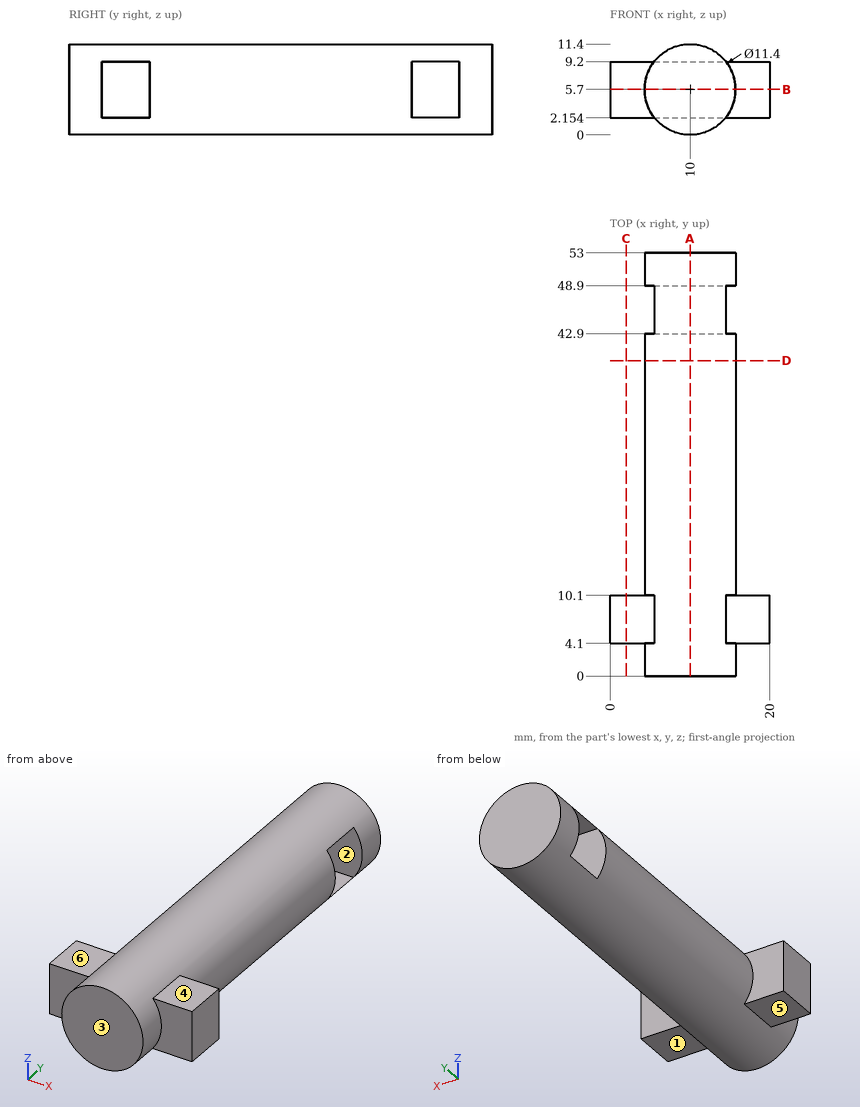
Part print with two shaded views. Sizes in mm from the minimum x, y, z corner. A direction names the side the tool comes from. Give positions to 0.01 mm unless a question says otherwise; leave off trailing zeros. Order: outer loops, then holes, each group sorted by start corner. A loop starts at its lowest first (then second) coordinate and runs counter-clockwise, first axis right, second up. Notation, with made-up numbers: (86.5, 19.5) - (123.5, 19.5) arc R11 ccw to (123.5, 35.5) - close; hole circle Ø2 at (-22.5, 44.25). An arc over 180 degrees is marked (long way). Write each question's results on one line, items separated by ' | '.
1. 3-axis set-ups, long thin cutter, end or side, ignore diameter. For the marked faces 4, 5 and 6: which of +Z, -Z, +X, -X, +Y, -Y reach the whole face in a straight line?
Calculated:
face 4: +Z, +X, +Y, -Y | face 5: -Z, -X, +Y, -Y | face 6: +Z, -X, +Y, -Y
2. Saw through at D-D on y = 39.5. List the corners of the cut face in (x, z), and give its area (3 significant figures).
Calculated:
outline: circle Ø11.4 at (10, 5.7) | area: 102 mm2
3. Pin check, flat tips, straight feed: pin 1 (4.5 mm diameter, centred on x = 4, y = 7, fed in from +Z); pin 2 (6 mm diameter, centred on y = 46.5, z = 7.5, fed in from +X); pin 3 (1.8 mm diameter, centred on x = 8, y = 44.5, fed in from -Z). Stop position of each tip, or through.
Calculated:
pin 1: stops at z = 9.99 | pin 2: stops at x = 15.7 | pin 3: stops at z = 0.11
4. Saw through at C-C on x = 2. List the corners of the cut face in (y, z) (1 decimal).
Calculated:
outline: (4.1, 2.2) - (10.1, 2.2) - (10.1, 9.2) - (4.1, 9.2) - close
5. Pull direction Z, two halves, no side cores. Call the marked faces 1, 2 and 3: released by +Z, released by -Z, zero draft, split by the parting line, or undercut.
Calculated:
face 1: released by -Z | face 2: undercut | face 3: zero draft
6. Saw through at B-B on z = 5.7. List the corners of the cut face in (x, y).
Calculated:
outline: (0, 4.1) - (4.3, 4.1) - (4.3, 0) - (15.7, 0) - (15.7, 4.1) - (20, 4.1) - (20, 10.1) - (15.7, 10.1) - (15.7, 42.9) - (4.3, 42.9) - (4.3, 10.1) - (0, 10.1) - close; (4.3, 48.9) - (15.7, 48.9) - (15.7, 53) - (4.3, 53) - close
7. Probe L1, parallel to Z at x = 3.5, y = 8.5 (1 decimal); L2, parallel to X at y = 12.5, z = 6; L3, parallel to Y at x = 2.5, z = 5.5. List the from-to ranges inside material, lowest first. Write a range as from..to.
Calculated:
L1: z = 2.2..9.2 | L2: x = 4.31..15.69 | L3: y = 4.1..10.1
8. Saw through at A-A on x = 10. List the corners of the cut face in (y, z) (1 decimal).
Calculated:
outline: (0, 0) - (53, 0) - (53, 11.4) - (0, 11.4) - close; hole (42.9, 2.2) - (48.9, 2.2) - (48.9, 9.2) - (42.9, 9.2) - close
